from build123d import *

# Parameters (mm, degrees)
SKETCH1_R           = 32.5
BOSS_EXTRUDE1_DEPTH = 35
CUT_EXTRUDE2_START  = -30
SKETCH2_R           = 32.5
SKETCH2_R_2         = 30.5
CUT_EXTRUDE2_DEPTH  = 30
SKETCH3_R           = 28
SKETCH3_R_2         = 24
CUT_EXTRUDE3_DEPTH  = 25
SKETCH4_R           = 18
CUT_EXTRUDE4_DEPTH  = 20
SKETCH5_R           = 0.5
CUT_EXTRUDE5_DEPTH  = 58.771100041
SKETCH6_R           = 2
CUT_EXTRUDE6_DEPTH  = 58.771100041


with BuildPart() as part:
    # Sketch1 → Boss-Extrude1 (new body)
    with BuildSketch(Plane(origin=(0, 0, 0), x_dir=(1, 0, 0), z_dir=(0, 1, 0))):
        with Locations(Location((0, 0, 0), (0, 0, 270))):
            Circle(SKETCH1_R)
    extrude(amount=BOSS_EXTRUDE1_DEPTH)

    # Sketch2 → Cut-Extrude2 (cut)
    with BuildSketch(Plane(origin=(0, 35, 0), x_dir=(1, 0, 0), z_dir=(0, 1, 0)).offset(CUT_EXTRUDE2_START)):
        with Locations(Location((0, 0, 0), (0, 0, 270))):
            Circle(SKETCH2_R)
        with Locations(Location((0, 0, 0), (0, 0, 270))):
            Circle(SKETCH2_R_2, mode=Mode.SUBTRACT)
    extrude(amount=CUT_EXTRUDE2_DEPTH, mode=Mode.SUBTRACT)

    # Sketch3 → Cut-Extrude3 (cut)
    with BuildSketch(Plane.XZ):
        with Locations(Location((0, 0, 0), (0, 0, 270))):
            Circle(SKETCH3_R)
        with Locations(Location((0, 0, 0), (0, 0, 270))):
            Circle(SKETCH3_R_2, mode=Mode.SUBTRACT)
    extrude(amount=-CUT_EXTRUDE3_DEPTH, mode=Mode.SUBTRACT)

    # Sketch4 → Cut-Extrude4 (cut)
    with BuildSketch(Plane.XZ):
        with Locations(Location((0, 0, 0), (0, 0, 270))):
            Circle(SKETCH4_R)
    extrude(amount=-CUT_EXTRUDE4_DEPTH, mode=Mode.SUBTRACT)

    # Sketch5 → Cut-Extrude5 (cut, through all)
    with BuildSketch(Plane(origin=(0, 35, 0), x_dir=(1, 0, 0), z_dir=(0, 1, 0))):
        with Locations(Location((-26, 0, 0), (0, 0, 270))):
            Circle(SKETCH5_R)
        with Locations(Location((26, 0, 0), (0, 0, 270))):
            Circle(SKETCH5_R)
    extrude(amount=-CUT_EXTRUDE5_DEPTH, mode=Mode.SUBTRACT)

    # Sketch6 → Cut-Extrude6 (cut, through all)
    with BuildSketch(Plane(origin=(0, 35, 0), x_dir=(1, 0, 0), z_dir=(0, 1, 0))):
        with Locations(Location((0, 0, 0), (0, 0, 270))):
            Circle(SKETCH6_R)
    extrude(amount=-CUT_EXTRUDE6_DEPTH, mode=Mode.SUBTRACT)


solid = part.part
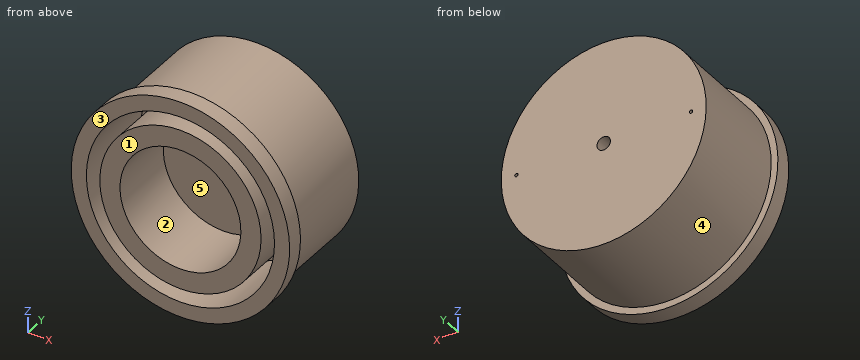
Build history of the part. All positions in model axes, mm. Face numbers are marked on the shaded views. A direction names the side the tool comes from. Coordinates: 2 decimals unless noted, no trailing zeros. Write each loop counter-clockwise with the first axis right and the second up, starting at its lowest first coordinate (ties: lowest second). Pieces come first, ordered by that corner, then holes.
(1) Cut at B-B on y = 7. List the corners of the cut face in (x, z), and give its area (3 significant figures).
(2) 3-axis set-ups, long thin cutter, end or side, ignore diameter. For the marked faces 1 and 2: which of +Z, -Z, +X, -X, +Y, -Y reach the whole face in a straight line?
(3) Mould opens along X. For the marked faces 3, 4 and 5 say: pulls with the +X half, pulls with the -X half, needs draft (parallel to the pull), parting line crosses it, or undercut.
(4) Cut at A-A on x = 0. List the corners of the cut face in (y, z), and give its area (4 significant figures).
(5) Pin check, flat tips, straight feed: pin 1 Ø21.5 at (x, z) = (0, 0) entering from -Y; pin 2 Ø1 at (x, y) = (12, 23) entering from -Z; pin 3 Ø8 at (y, z) = (28, 13) entering from +X; pin 4 Ø2.5 at (x, z) = (0, 0) entering from -Y. Stop position of each tip, or through.
(6) Cut at D-D on y = 33.5. List the corners of the cut face in (x, z), and give its area (3 significant figures).
(7) Drill centre lines: line 1 (X direction, y = 18.5, z = 0); line 2 (X direction, y = 23.75, z = 0); line 3 (Z direction, x = -6, y = 9). Where is each one in solid material? Low to high.
(8) Cut at C-C on z = -6. List the corners of the cut face in (x, y), and give its area (3 significant figures).
Working result:
1. outline: circle Ø61 at (0, 0); circle Ø48 at (0, 0); hole circle Ø56 at (0, 0); hole circle Ø36 at (0, 0)
1. area: 1,250 mm2
2. face 1: +Z, -Z, +X, -X, -Y
2. face 2: -Y
3. face 3: needs draft
3. face 4: parting line crosses it
3. face 5: undercut
4. outline: (0, -32.5) - (5, -32.5) - (5, -30.5) - (35, -30.5) - (35, -2) - (20, -2) - (20, -18) - (0, -18) - (0, -24) - (25, -24) - (25, -28) - (0, -28) - close; (0, 18) - (20, 18) - (20, 2) - (35, 2) - (35, 30.5) - (5, 30.5) - (5, 32.5) - (0, 32.5) - (0, 28) - (25, 28) - (25, 24) - (0, 24) - close
4. area: 1,175 mm2
5. pin 1: stops at y = 20
5. pin 2: stops at z = -28.25
5. pin 3: stops at x = 29.14
5. pin 4: passes through
6. outline: circle Ø61 at (0, 0); hole circle Ø1 at (-26, 0); hole circle Ø4 at (0, 0); hole circle Ø1 at (26, 0)
6. area: 2,910 mm2
7. line 1: x = -30.5 to -28, -24 to -18, 18 to 24, 28 to 30.5
7. line 2: x = -30.5 to -28, -24 to -2, 2 to 24, 28 to 30.5
7. line 3: z = -29.9 to -27.35, -23.24 to -16.97, 16.97 to 23.24, 27.35 to 29.9
8. outline: (-31.94, 0) - (-27.35, 0) - (-27.35, 25) - (-23.24, 25) - (-23.24, 0) - (-16.97, 0) - (-16.97, 20) - (16.97, 20) - (16.97, 0) - (23.24, 0) - (23.24, 25) - (27.35, 25) - (27.35, 0) - (31.94, 0) - (31.94, 5) - (29.9, 5) - (29.9, 35) - (-29.9, 35) - (-29.9, 5) - (-31.94, 5) - close
8. area: 1,230 mm2
